from build123d import *
from OCP.BRepFilletAPI import BRepFilletAPI_MakeChamfer

# Parameters (mm, degrees)
SKETCH1_R           = 98
BOSS_EXTRUDE1_DEPTH = 24
FILLET1_R           = 12
CHAMFER1_SIZE       = 3
CHAMFER1_SIZE2      = 1.732050808
CHAMFER2_SIZE       = 3
CHAMFER2_SIZE2      = 1.732050808


with BuildPart() as part:
    # Sketch1 → Boss-Extrude1 (new body)
    with BuildSketch(Plane(origin=(0, 0, 0), x_dir=(1, 0, 0), z_dir=(0, 1, 0))):
        with Locations(Location((0, 0, 0), (0, 0, 270))):
            Circle(SKETCH1_R)
        with BuildLine():
            Line((-73.020545054, 12), (73.020545054, 12))
            ThreePointArc((73.020545054, 12), (0, 74), (-73.020545054, 12))
        make_face(mode=Mode.SUBTRACT)
        with BuildLine():
            Line((73.020545054, -12), (-73.020545054, -12))
            ThreePointArc((-73.020545054, -12), (0, -74), (73.020545054, -12))
        make_face(mode=Mode.SUBTRACT)
    extrude(amount=BOSS_EXTRUDE1_DEPTH)

    # Fillet1
    fillet1_edges = [part.edges().sort_by_distance(p)[0] for p in [
        (-73.020545054, 12, 12),
        (73.020545054, 12, 12),
        (73.020545054, 12, -12),
        (-73.020545054, 12, -12),
    ]]
    fillet(fillet1_edges, radius=FILLET1_R)

    # Chamfer1: one chamfer whose edges measure the first distance from different faces: ONE call of the kernel's chamfer builder (chamfer() names one face for all edges)
    chamfer1_edges_1 = [part.edges().sort_by_distance(p)[0] for p in [
        (0, 0, 74),
    ]]
    chamfer1_side_1 = [part.faces().sort_by_distance(p)[0] for p in [
        (0, 12, 74),
    ]]
    chamfer1_edges_2 = [part.edges().sort_by_distance(p)[0] for p in [
        (0, 0, 12),
    ]]
    chamfer1_side_2 = [part.faces().sort_by_distance(p)[0] for p in [
        (0, 12, 12),
    ]]
    chamfer1_edges_3 = [part.edges().sort_by_distance(p)[0] for p in [
        (0, 0, -12),
    ]]
    chamfer1_side_3 = [part.faces().sort_by_distance(p)[0] for p in [
        (0, 12, -12),
    ]]
    chamfer1_edges_4 = [part.edges().sort_by_distance(p)[0] for p in [
        (0, 0, -74),
    ]]
    chamfer1_side_4 = [part.faces().sort_by_distance(p)[0] for p in [
        (0, 12, -74),
    ]]
    chamfer1_edges_5 = [part.edges().sort_by_distance(p)[0] for p in [
        (67.159970016, 0, 17.357031367),
    ]]
    chamfer1_side_5 = [part.faces().sort_by_distance(p)[0] for p in [
        (67.159970016, 12, 17.357031367),
    ]]
    chamfer1_edges_6 = [part.edges().sort_by_distance(p)[0] for p in [
        (67.159970016, 0, -17.357031367),
    ]]
    chamfer1_side_6 = [part.faces().sort_by_distance(p)[0] for p in [
        (67.159970016, 12, -17.357031367),
    ]]
    chamfer1_edges_7 = [part.edges().sort_by_distance(p)[0] for p in [
        (-67.159970016, 0, -17.357031367),
    ]]
    chamfer1_side_7 = [part.faces().sort_by_distance(p)[0] for p in [
        (-67.159970016, 12, -17.357031367),
    ]]
    chamfer1_edges_8 = [part.edges().sort_by_distance(p)[0] for p in [
        (-67.159970016, 0, 17.357031367),
    ]]
    chamfer1_side_8 = [part.faces().sort_by_distance(p)[0] for p in [
        (-67.159970016, 12, 17.357031367),
    ]]
    chamfer1_edges_9 = [part.edges().sort_by_distance(p)[0] for p in [
        (0, 24, -98),
    ]]
    chamfer1_side_9 = [part.faces().sort_by_distance(p)[0] for p in [
        (0, 12, -98),
    ]]
    chamfer1 = BRepFilletAPI_MakeChamfer(part.part.solid().wrapped)
    for e in chamfer1_edges_1:
        chamfer1.Add(CHAMFER1_SIZE, CHAMFER1_SIZE2, e.wrapped, chamfer1_side_1[0].wrapped)  # the first distance lies on this face
    for e in chamfer1_edges_2:
        chamfer1.Add(CHAMFER1_SIZE, CHAMFER1_SIZE2, e.wrapped, chamfer1_side_2[0].wrapped)  # the first distance lies on this face
    for e in chamfer1_edges_3:
        chamfer1.Add(CHAMFER1_SIZE, CHAMFER1_SIZE2, e.wrapped, chamfer1_side_3[0].wrapped)  # the first distance lies on this face
    for e in chamfer1_edges_4:
        chamfer1.Add(CHAMFER1_SIZE, CHAMFER1_SIZE2, e.wrapped, chamfer1_side_4[0].wrapped)  # the first distance lies on this face
    for e in chamfer1_edges_5:
        chamfer1.Add(CHAMFER1_SIZE, CHAMFER1_SIZE2, e.wrapped, chamfer1_side_5[0].wrapped)  # the first distance lies on this face
    for e in chamfer1_edges_6:
        chamfer1.Add(CHAMFER1_SIZE, CHAMFER1_SIZE2, e.wrapped, chamfer1_side_6[0].wrapped)  # the first distance lies on this face
    for e in chamfer1_edges_7:
        chamfer1.Add(CHAMFER1_SIZE, CHAMFER1_SIZE2, e.wrapped, chamfer1_side_7[0].wrapped)  # the first distance lies on this face
    for e in chamfer1_edges_8:
        chamfer1.Add(CHAMFER1_SIZE, CHAMFER1_SIZE2, e.wrapped, chamfer1_side_8[0].wrapped)  # the first distance lies on this face
    for e in chamfer1_edges_9:
        chamfer1.Add(CHAMFER1_SIZE, CHAMFER1_SIZE2, e.wrapped, chamfer1_side_9[0].wrapped)  # the first distance lies on this face
    add(Compound.cast(chamfer1.Shape()), mode=Mode.REPLACE)

    # Chamfer2: one chamfer whose edges measure the first distance from different faces: ONE call of the kernel's chamfer builder (chamfer() names one face for all edges)
    chamfer2_edges_1 = [part.edges().sort_by_distance(p)[0] for p in [
        (0, 0, -98),
    ]]
    chamfer2_side_1 = [part.faces().sort_by_distance(p)[0] for p in [
        (0, 10.5, -98),
    ]]
    chamfer2_edges_2 = [part.edges().sort_by_distance(p)[0] for p in [
        (0, 24, 74),
    ]]
    chamfer2_side_2 = [part.faces().sort_by_distance(p)[0] for p in [
        (0, 13.5, 74),
    ]]
    chamfer2_edges_3 = [part.edges().sort_by_distance(p)[0] for p in [
        (0, 24, 12),
    ]]
    chamfer2_side_3 = [part.faces().sort_by_distance(p)[0] for p in [
        (0, 13.5, 12),
    ]]
    chamfer2_edges_4 = [part.edges().sort_by_distance(p)[0] for p in [
        (0, 24, -12),
    ]]
    chamfer2_side_4 = [part.faces().sort_by_distance(p)[0] for p in [
        (0, 13.5, -12),
    ]]
    chamfer2_edges_5 = [part.edges().sort_by_distance(p)[0] for p in [
        (0, 24, -74),
    ]]
    chamfer2_side_5 = [part.faces().sort_by_distance(p)[0] for p in [
        (0, 13.5, -74),
    ]]
    chamfer2_edges_6 = [part.edges().sort_by_distance(p)[0] for p in [
        (67.159970016, 24, 17.357031367),
    ]]
    chamfer2_side_6 = [part.faces().sort_by_distance(p)[0] for p in [
        (67.159970016, 13.5, 17.357031367),
    ]]
    chamfer2_edges_7 = [part.edges().sort_by_distance(p)[0] for p in [
        (67.159970016, 24, -17.357031367),
    ]]
    chamfer2_side_7 = [part.faces().sort_by_distance(p)[0] for p in [
        (67.159970016, 13.5, -17.357031367),
    ]]
    chamfer2_edges_8 = [part.edges().sort_by_distance(p)[0] for p in [
        (-67.159970016, 24, -17.357031367),
    ]]
    chamfer2_side_8 = [part.faces().sort_by_distance(p)[0] for p in [
        (-67.159970016, 13.5, -17.357031367),
    ]]
    chamfer2_edges_9 = [part.edges().sort_by_distance(p)[0] for p in [
        (-67.159970016, 24, 17.357031367),
    ]]
    chamfer2_side_9 = [part.faces().sort_by_distance(p)[0] for p in [
        (-67.159970016, 13.5, 17.357031367),
    ]]
    chamfer2 = BRepFilletAPI_MakeChamfer(part.part.solid().wrapped)
    for e in chamfer2_edges_1:
        chamfer2.Add(CHAMFER2_SIZE, CHAMFER2_SIZE2, e.wrapped, chamfer2_side_1[0].wrapped)  # the first distance lies on this face
    for e in chamfer2_edges_2:
        chamfer2.Add(CHAMFER2_SIZE, CHAMFER2_SIZE2, e.wrapped, chamfer2_side_2[0].wrapped)  # the first distance lies on this face
    for e in chamfer2_edges_3:
        chamfer2.Add(CHAMFER2_SIZE, CHAMFER2_SIZE2, e.wrapped, chamfer2_side_3[0].wrapped)  # the first distance lies on this face
    for e in chamfer2_edges_4:
        chamfer2.Add(CHAMFER2_SIZE, CHAMFER2_SIZE2, e.wrapped, chamfer2_side_4[0].wrapped)  # the first distance lies on this face
    for e in chamfer2_edges_5:
        chamfer2.Add(CHAMFER2_SIZE, CHAMFER2_SIZE2, e.wrapped, chamfer2_side_5[0].wrapped)  # the first distance lies on this face
    for e in chamfer2_edges_6:
        chamfer2.Add(CHAMFER2_SIZE, CHAMFER2_SIZE2, e.wrapped, chamfer2_side_6[0].wrapped)  # the first distance lies on this face
    for e in chamfer2_edges_7:
        chamfer2.Add(CHAMFER2_SIZE, CHAMFER2_SIZE2, e.wrapped, chamfer2_side_7[0].wrapped)  # the first distance lies on this face
    for e in chamfer2_edges_8:
        chamfer2.Add(CHAMFER2_SIZE, CHAMFER2_SIZE2, e.wrapped, chamfer2_side_8[0].wrapped)  # the first distance lies on this face
    for e in chamfer2_edges_9:
        chamfer2.Add(CHAMFER2_SIZE, CHAMFER2_SIZE2, e.wrapped, chamfer2_side_9[0].wrapped)  # the first distance lies on this face
    add(Compound.cast(chamfer2.Shape()), mode=Mode.REPLACE)


solid = part.part
Design review of the part built by this model. Coordinates are the model's own, in mm. A direction names the side the tool comes from. Give positions to 0.01 mm unless a question says otherwise; leave off trailing zeros. Loops run counter-clockwise (first coordinate to the right, second up) from the corner with the lowest first, then second, coordinate; pieces in that order, holes last. Notation, with made-up numbers: M -33,-16.75 L -14,-16.75 A31 ccw -14,15.25 Z; hole C 54,-37.75 d2. An arc over 180 degrees is marked long. Answer as a JSON object with one key per item and string values.
Item 1: Wall thickness on line 1 along Z through (x, y) = (54.5, 15); line 2 along Z through (x, y) = (-43, 10.25); line 3 along X through (y, z) = (2.25, -55): over which ranges is each line inside the solid? List them lowest first.
Output values:
{"line 1": "z = -81.45 to -50.06, -12 to 12, 50.06 to 81.45", "line 2": "z = -88.06 to -60.22, -12 to 12, 60.22 to 88.06", "line 3": "x = -80.59 to -50.15, 50.15 to 80.59"}
Item 2: For P1, Ø3, axis at y = 19.5, z = 38, coming from the -X side; P2, Ø6, axis at y = 8, z = -44.5, coming from the +X side; P3, Ø1.5, axis at x = -74, y = 17, coming from the +Z side, all flat-tipped, find the tip position at first contact; note any pin that passes through.
Output values:
{"P1": "stops at x = -90.95", "P2": "stops at x = 88.78", "P3": "stops at z = 65.1"}
Item 3: Machinability: for faces 1 (the face through (1, 0, -1)), 2 (the face through (1.22, 11.87, -73.99)), which of the approach directions +Z, -Z, +X, -X, +Y, -Y give a long, thin tool a straight path to every point of the face, cutting with its end or side? Answer none if there is none.
Output values:
{"face 1": "+Z, -Z, +X, -X, -Y", "face 2": "+Y, -Y"}
Item 4: We need section C-C (x = -63). Count the separate pieces of the cut face and the enclosed holes in it, and give its area (3 significant figures).
Output values:
{"separate pieces": "3", "enclosed holes": "0", "area": "2,340 mm2"}
Item 5: Mouldability with a two-part tool opening along X and no side actions: class faces 3 (the face through (67.067, 12.126, -17.22)), 4 (the face through (-94.061, 23.854, -20.887)), 5 (the face through (1, 24, -1)) as pulls with the +X half, pulls with the -X half, needs draft (parallel to the pull), parting line crosses it, or undercut.
Output values:
{"face 3": "undercut", "face 4": "parting line crosses it", "face 5": "needs draft"}
Item 6: We need section A-A (y = 11.5). State the section outline as (x, z) points, and give its area (3 significant figures).
Output values:
{"outline": "C 0,0 d196; hole M -68.23,-28.65 A74 ccw 68.23,-28.65 A12 ccw 57.17,-12 L -57.17,-12 A12 ccw Z; hole M -68.23,28.65 A12 ccw -57.17,12 L 57.17,12 A12 ccw 68.23,28.65 A74 ccw Z", "area": "16,800 mm2"}
Item 7: We need section B-B (x = 0). State the section outline as (y, z) points, and give its area (3 significant figures).
Output values:
{"outline": "M 0,-96.27 L 3,-98 L 21,-98 L 24,-96.27 L 24,-75.73 L 21,-74 L 3,-74 L 0,-75.73 Z; M 0,-10.27 L 3,-12 L 21,-12 L 24,-10.27 L 24,10.27 L 21,12 L 3,12 L 0,10.27 Z; M 0,75.73 L 3,74 L 21,74 L 24,75.73 L 24,96.27 L 21,98 L 3,98 L 0,96.27 Z", "area": "1,700 mm2"}
